Drawing for the job (mm, zero at the part's lowest x, y, z). A direction names the side the tool comes from. Coordinates: 2 decimals unless noted, no trailing zeros. Order: outer loops, then holes, each group sorted by start corner. A loop starts at its lowest first (then second) coordinate and runs counter-clockwise, first axis right, second up.
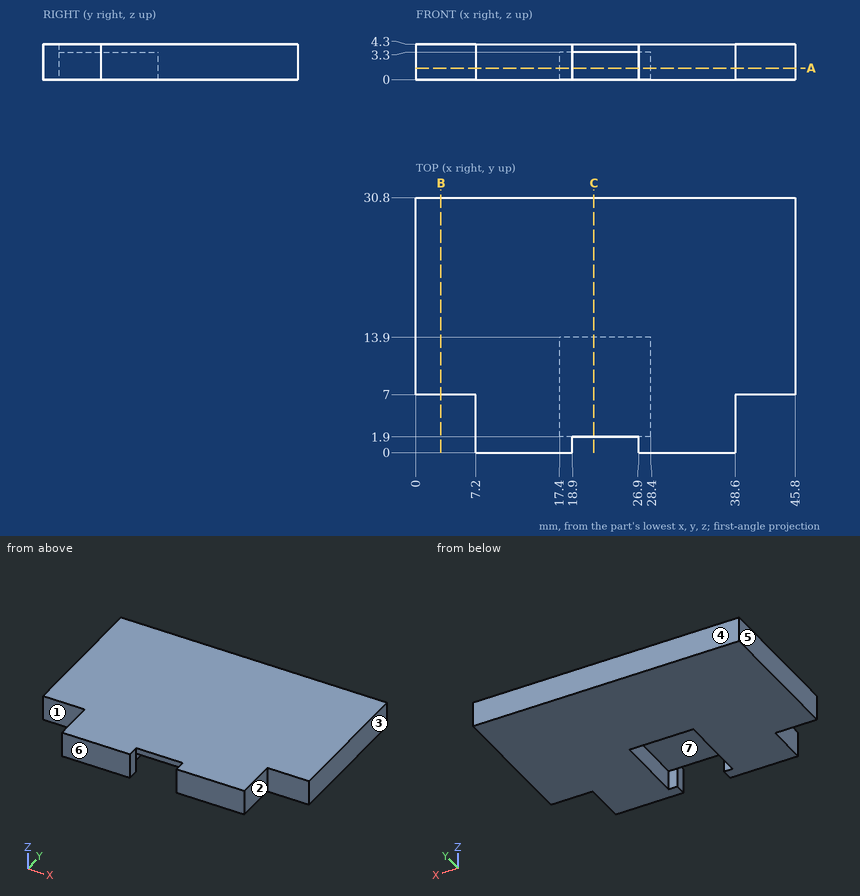
(1) Slice it at A-A, the plane z = 1.4. Give the cut face in (x, y).
(2) Drop flat-ended pins along their axis: pin 1 (1.1 mm diameter, centred on x = 21, z = 4, fed in from -Y); pin 2 (1.3 mm diameter, centred on x = 5.5, z = 2, fed in from -Y); pin 3 (2 mm diameter, centred on y = 0.5, z = 1.5, fed in from -X). Give the stop position or say it passes through.
(3) Slice it at B-B, the plane x = 3. Give the cut face in (y, z), then the cut area to 3 significant figures.
(4) Tool access for the marked faces 1, 2 and 3: list every direction of +Z, -Z, +X, -X, +Y, -Y with a clear straight run to the whole face (end or side of a thin tool).
(5) Pull direction Y, two halves, no side cores. Call the marked faces 4, 5, 6 and 7: +Y half, -Y half, draft (parallel to the pull), parting line (faces both ways), or undercut.
(6) Slice it at C-C, the plane x = 21.5. Give the cut face in (y, z).
(7) Probe line 1 (X direction, y = 8.5, z = 1.8); line 2 (X direction, y = 2.5, z = 1.25); line 3 (Y direction, x = 2, z = 3.7). List the from-to ranges inside material, lowest first.
Here are the results:
1. outline: (0, 7) - (7.2, 7) - (7.2, 0) - (18.9, 0) - (18.9, 1.9) - (17.4, 1.9) - (17.4, 13.9) - (28.4, 13.9) - (28.4, 1.9) - (26.9, 1.9) - (26.9, 0) - (38.6, 0) - (38.6, 7) - (45.8, 7) - (45.8, 30.8) - (0, 30.8) - close
2. pin 1: stops at y = 1.9
2. pin 2: stops at y = 7
2. pin 3: stops at x = 7.2
3. outline: (7, 0) - (30.8, 0) - (30.8, 4.3) - (7, 4.3) - close
3. area: 102 mm2
4. face 1: +Z, -Z, -X, -Y
4. face 2: +Z, -Z, +X, -Y
4. face 3: +Z, -Z, +X, +Y, -Y
5. face 4: +Y half
5. face 5: draft
5. face 6: -Y half
5. face 7: undercut
6. outline: (1.9, 3.3) - (13.9, 3.3) - (13.9, 0) - (30.8, 0) - (30.8, 4.3) - (1.9, 4.3) - close
7. line 1: x = 0 to 17.4, 28.4 to 45.8
7. line 2: x = 7.2 to 17.4, 28.4 to 38.6
7. line 3: y = 7 to 30.8
